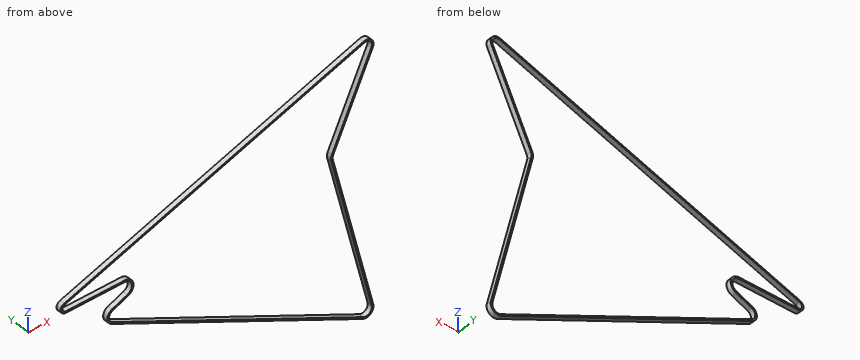
from build123d import *

# Parameters (mm, degrees)
EXTRUDE_THIN1_DEPTH = 6


with BuildPart() as part:
    # Sketch1 → Extrude-Thin1 (new body)
    with BuildSketch(Plane(origin=(0, 86.8, 0), x_dir=(1, 0, 0), z_dir=(0, 1, 0))):
        with BuildLine():
            Line((153.976470843, 166.722058314), (-162.473529157, 8.497058315))
            ThreePointArc((-162.473529157, 8.497058314), (-167.715732066, -0.419529316), (-161.707213549, -8.838788876))
            Line((-161.707213549, -8.838788876), (-142.250173329, -16.504269977))
            ThreePointArc((-142.250173329, -16.504269977), (-136.846395058, -26.198255989), (-145.296171508, -33.393772811))
            Line((-145.296171508, -33.393772811), (-220.267521321, -34.776083328))
            ThreePointArc((-220.267521321, -34.776083328), (-226.458318107, -40.230354602), (-222.082372691, -47.225077019))
            Line((-222.082372691, -47.225077019), (155.345385794, -167.278055949))
            ThreePointArc((155.345385794, -167.278055949), (165.396500417, -164.455536235), (166.786864342, -154.108632792))
            Line((166.786864342, -154.108632792), (117.114072317, -50.79139085))
            ThreePointArc((117.114072317, -50.79139085), (116.29360588, -47.872468586), (116.518563148, -44.848784313))
            Line((116.518563148, -44.848784313), (167.433417153, 155.889394397))
            ThreePointArc((167.433417153, 155.889394397), (164.182077649, 165.625217962), (153.976470843, 166.722058314))
        make_face()
        with BuildLine():
            Line((154.870898034, 164.933203932), (-161.579101966, 6.708203933))
            ThreePointArc((-161.579101966, 6.708203933), (-165.71768321, -0.331207355), (-160.97411596, -6.977991218))
            Line((-160.97411596, -6.977991218), (-141.517075739, -14.643472319))
            ThreePointArc((-141.517075739, -14.643472319), (-134.87814815, -26.553226562), (-145.259302074, -35.393432943))
            Line((-145.259302074, -35.393432943), (-220.230651887, -36.775743461))
            ThreePointArc((-220.230651887, -36.775743461), (-224.479237917, -40.518870805), (-221.476138121, -45.319170503))
            Line((-221.476138121, -45.319170503), (155.951620364, -165.372149434))
            ThreePointArc((155.951620364, -165.372149434), (163.886710855, -163.143844396), (164.984366586, -154.975236414))
            Line((164.984366586, -154.975236414), (115.311574561, -51.657994473))
            ThreePointArc((115.311574561, -51.657994473), (114.303572939, -48.071889977), (114.579949011, -44.35707787))
            Line((114.579949011, -44.35707787), (165.494803016, 156.38110084))
            ThreePointArc((165.494803016, 156.38110084), (162.927956039, 164.067277338), (154.870898034, 164.933203932))
        make_face(mode=Mode.SUBTRACT)
    extrude(amount=EXTRUDE_THIN1_DEPTH)


solid = part.part
CAD build for the part. Positions are in the model's coordinates, mm. Give positions to 0.01 mm unless a question says otherwise; leave off trailing zeros. Write each loop counter-clockwise with the first axis right and the second up, starting at its lowest first coordinate (ties: lowest second). Pieces come first, ordered by that corner, then holes. Notation, with made-up numbers: (72, -5.5) - (85, -5.5) arc R17 cw to (85, 11.5) - close; hole circle Ø5 at (37.25, 45.5). An arc over 180 degrees is marked (long way). Answer as CSV lines item,"result".
Q1. Flat gauge pins, fed straight in: pin 1 Ø3 at (x, y) = (9, 91.5) entering from +Z; pin 2 Ø1.5 at (y, z) = (89, -71) entering from -X. Where does each tip first touch, or does it go through?
Result set:
pin 1,"z = 121.21"
pin 2,"x = -38.97"
Q2. Band-saw the part on A-A (x = -185.5). Give the cut face in (y, z), and give its area (3 significant figures).
Result set:
outline,"(86.8, 34.14) - (92.8, 34.14) - (92.8, 36.14) - (86.8, 36.14) - close; (86.8, 56.76) - (92.8, 56.76) - (92.8, 58.86) - (86.8, 58.86) - close"
area,"24.6 mm²"
Q3. Band-saw the part on B-B (y = 88.6). Give the cut face in (x, z) (3 decimals), and give its area (3 significant figures).
Result set:
outline,"(-222.082, 47.225) arc R6.375 ccw to (-220.268, 34.776) - (-145.296, 33.394) arc R8.75 cw to (-142.25, 16.504) - (-161.707, 8.839) arc R9.5 ccw to (-162.474, -8.497) - (153.976, -166.722) arc R9.5 ccw to (167.433, -155.889) - (116.519, 44.849) arc R8.75 cw to (117.114, 50.791) - (166.787, 154.109) arc R9.5 ccw to (155.345, 167.278) - close; hole (-221.476, 45.319) arc R4.375 ccw to (-220.231, 36.776) - (-145.259, 35.393) arc R10.75 cw to (-141.517, 14.643) - (-160.974, 6.978) arc R7.5 ccw to (-161.579, -6.708) - (154.871, -164.933) arc R7.5 ccw to (165.495, -156.381) - (114.58, 44.357) arc R10.75 cw to (115.312, 51.658) - (164.984, 154.975) arc R7.5 ccw to (155.952, 165.372) - close"
area,"2,550 mm²"
Q4. Drill centre lines: line 1 (Z direction, x = -155, y = 87.45); line 2 (Z direction, x = 12.5, y = 89.35); line 3 (Z direction, x = 20, y = 88.55). Where is each one in solid material? Low to high. Write a range as from..to.
Result set:
line 1,"-12.23..-10, 9.33..11.48, 33.57..35.57, 66.46..68.56"
line 2,"-95.98..-93.75, 119.74..121.84"
line 3,"-99.73..-97.5, 122.13..124.23"
Q5. Band-saw the part on D-D (x = 136.5). Give the cut face in (y, z).
Result set:
outline,"(86.8, -157.98) - (92.8, -157.98) - (92.8, -155.75) - (86.8, -155.75) - close; (86.8, -42.07) - (92.8, -42.07) - (92.8, -33.93) - (86.8, -33.93) - close; (86.8, 91.11) - (92.8, 91.11) - (92.8, 95.73) - (86.8, 95.73) - close; (86.8, 159.18) - (92.8, 159.18) - (92.8, 161.28) - (86.8, 161.28) - close"
Q6. Band-saw the part on C-C (z = 127.5). Give the cut face in (x, y).
Result set:
outline,"(30.29, 86.8) - (36.89, 86.8) - (36.89, 92.8) - (30.29, 92.8) - close; (151.77, 86.8) - (153.99, 86.8) - (153.99, 92.8) - (151.77, 92.8) - close"
